CAD build for the part. Positions are in the model's coordinates, mm. A direction names the side the tool comes from. Give positions to 0.01 mm unless a question says otherwise; leave off trailing zeros. Loops run counter-clockwise (first coordinate to the right, second up) from the corner with the lowest first, then second, coordinate; pieces in that order, holes last. Notation, with made-up numbers: (-13, -13.5) - (-8, -13.5) arc R22 ccw to (-8, -5.5) - close; hole circle Ø10 at (45, -20.5). An arc over 180 degrees is marked (long way). Return JSON: item names as keys, results as strings.
from build123d import *

# Parameters (mm, degrees)
EXTRUDE_1_DEPTH     = 14
SKETCH_3_W          = 6
SKETCH_3_H          = 12
CUT_EXTRUDE_1_DEPTH = 19.848076825
FILLET_2_R          = 1


with BuildPart() as part:
    # 草图2 → 凸台-拉伸1 (new body)
    with BuildSketch(Plane(origin=(0, 0, 0), x_dir=(0, 0, -1), z_dir=(1, 0, 0))):
        with BuildLine():
            Line((10.5, 0), (3, 0))
            Line((3, 0), (3, 2))
            ThreePointArc((3, 2), (0, 5), (-3, 2))
            Line((-3, 2), (-3, 0))
            Line((-3, 0), (-10.5, 0))
            Line((-10.5, 0), (-10.5, 3))
            Line((-10.5, 3), (-4.898979486, 3))
            ThreePointArc((-4.898979486, 3), (0, 7), (4.898979486, 3))
            Line((4.898979486, 3), (10.5, 3))
            Line((10.5, 3), (10.5, 0))
        make_face()
    extrude(amount=EXTRUDE_1_DEPTH)

    # 草图3 → 切除-拉伸1 (cut, through all)
    with BuildSketch(Plane.XZ):
        with Locations((7, 0)):
            Rectangle(SKETCH_3_W, SKETCH_3_H)
    extrude(amount=-CUT_EXTRUDE_1_DEPTH, mode=Mode.SUBTRACT)

    # 圆角2
    fillet_2_edges = [part.edges().sort_by_distance(p)[0] for p in [
        (12, 3, 4.898979486),
        (12, 3, -4.898979486),
        (2, 3, 4.898979486),
        (2, 3, -4.898979486),
    ]]
    fillet(fillet_2_edges, radius=FILLET_2_R)


solid = part.part
1. Pull direction Z, two halves, no side cores. Call faces 1 (the face through (7, 0, -7)), 2 (the face through (2, 5, 0)), 3 (the face through (7, 2, -10.5)): +Z half, -Z half, draft (parallel to the pull), parting line (faces both ways), or undercut.
Values follow:
{"face 1": "draft", "face 2": "undercut", "face 3": "-Z half"}
2. Drill centre lines: probe 1 along X at (y, z) = (5.75, -2.25); probe 2 along Z at (x, y) = (9, 2); probe 3 along Y at (x, z) = (5.25, -9.5). Where is each one in solid material? Low to high.
Values follow:
{"probe 1": "x = 0 to 4, 10 to 14", "probe 2": "z = -10.5 to -6, 6 to 10.5", "probe 3": "y = 0 to 3"}
3. Cut at D-D, the plane y = 4.5. Write the cut outline in (x, z).
Values follow:
{"outline": "(0, -4.33) - (4, -4.33) - (4, -1.66) - (0, -1.66) - close; (0, 1.66) - (4, 1.66) - (4, 4.33) - (0, 4.33) - close; (10, -4.33) - (14, -4.33) - (14, -1.66) - (10, -1.66) - close; (10, 1.66) - (14, 1.66) - (14, 4.33) - (10, 4.33) - close"}
4. Cut at C-C, the plane y = 2.75. Write the cut outline in (x, z), plus the area to 3 significant figures.
Values follow:
{"outline": "(0, -10.5) - (14, -10.5) - (14, -2.9) - (10, -2.9) - (10, -6) - (4, -6) - (4, -2.9) - (0, -2.9) - close; (0, 2.9) - (4, 2.9) - (4, 6) - (10, 6) - (10, 2.9) - (14, 2.9) - (14, 10.5) - (0, 10.5) - close", "area": "176 mm²"}
5. Cut at B-B, the plane z = 0. Write the cut outline in (x, y), plus the area to 3 significant figures.
Values follow:
{"outline": "(0, 5) - (4, 5) - (4, 7) - (0, 7) - close; (10, 5) - (14, 5) - (14, 7) - (10, 7) - close", "area": "16.0 mm²"}
6. Which spindle directions (+Z, -Z, +X, -X, +Y, -Y) get a long thin tool onto all of the face, cutting with end or side? Do faces 4 (the face through (7, 1, 6)), 5 (the face through (12, 1, 3)), 6 (the face through (7, 3, 8)), 7 (the face through (14, 4.3, 2.2)), 8 (the face through (2, 7, 0)). Say none if no direction does.
Values follow:
{"face 4": "+Y, -Y", "face 5": "+X, -X, -Y", "face 6": "+Z, +X, -X, +Y", "face 7": "+Z, -Z, +X, +Y, -Y", "face 8": "+X, -X, +Y"}
7. Drop flat-ended pins along their axis: P1, Ø5.5, axis at x = 5, z = 8, coming from the +Y side; P2, Ø4, axis at x = 10.5, y = 5.5, coming from the +Z side. Give the stop position or say it passes through.
Values follow:
{"P1": "stops at y = 3.02", "P2": "stops at z = 4.79"}
8. Cut at A-A, the plane x = 9.5. Write the cut outline in (y, z), plus the area to 3 significant figures.
Values follow:
{"outline": "(0, -10.5) - (3, -10.5) - (3, -6) - (0, -6) - close; (0, 6) - (3, 6) - (3, 10.5) - (0, 10.5) - close", "area": "27.0 mm²"}
